Work out the finished part from the listing and answer in its coordinate system (mm). Round coordinates to 2 decimals unless told otherwise and drop trailing zeros. Answer in a Markdown table with one row per item.
```python
from build123d import *

# Parameters (mm, degrees)
SKETCH1_R           = 1.65
SKETCH1_R_2         = 4.5
SKETCH1_R_3         = 2.2
SKETCH1_R_4         = 1.15
SKETCH1_W           = 22
SKETCH1_H           = 43
SKETCH1_W_2         = 40
SKETCH1_H_2         = 12
BOSS_EXTRUDE1_DEPTH = 3
FILLET2_R           = 3
FILLET3_R           = 2
FILLET4_R           = 10
SKETCH2_W           = 40
SKETCH2_H           = 3
BOSS_EXTRUDE2_DEPTH = 3
SKETCH3_W           = 40
SKETCH3_H           = 3
CUT_EXTRUDE1_DEPTH  = 3
FILLET5_R           = 3


with BuildPart() as part:
    # Sketch1 → Boss-Extrude1 (new body)
    with BuildSketch(Plane.XY):
        with BuildLine():
            Line((-65.69, -25.08927508), (-65.69, -107.741221405))
            Line((-65.69, -107.741221405), (-40.69, -107.741221405))
            Line((-40.69, -107.741221405), (-40.69, -164.982205675))
            Line((-40.69, -164.982205675), (40.69, -164.982205675))
            Line((40.69, -164.982205675), (40.69, -107.741221405))
            Line((40.69, -107.741221405), (65.69, -107.741221405))
            Line((65.69, -107.741221405), (65.69, -25.08927508))
            Line((65.69, -25.08927508), (28.641763355, 5.396592354))
            Line((28.641763355, 5.396592354), (28.641763355, 14.771578959))
            ThreePointArc((28.641763355, 14.771578959), (36.853483101, 20.369604934), (30.2775665, 27.821286413))
            Line((30.2775665, 27.821286413), (30.2775665, 37.695580673))
            Line((30.2775665, 37.695580673), (9.5975665, 65.017794325))
            Line((9.5975665, 65.017794325), (-9.5975665, 65.017794325))
            Line((-9.5975665, 65.017794325), (-30.2775665, 37.695580673))
            Line((-30.2775665, 37.695580673), (-30.2775665, 27.821286413))
            ThreePointArc((-30.2775665, 27.821286413), (-36.853483101, 20.369604934), (-28.641763355, 14.771578959))
            Line((-28.641763355, 14.771578959), (-28.641763355, 5.396592354))
            Line((-28.641763355, 5.396592354), (-65.69, -25.08927508))
        make_face()
        with Locations((-30.2775665, 21.193907325)):
            Circle(SKETCH1_R, mode=Mode.SUBTRACT)
        with Locations((-29.8216785, -158.982205675)):
            Circle(SKETCH1_R, mode=Mode.SUBTRACT)
        with Locations((-52.692806, -67.094311675)):
            Circle(SKETCH1_R, mode=Mode.SUBTRACT)
        with Locations(Location((30.2775665, 21.193907325, 0), (0, 0, 180))):
            Circle(SKETCH1_R, mode=Mode.SUBTRACT)
        with Locations(Location((52.692806, -67.094311675, 0), (0, 0, 180))):
            Circle(SKETCH1_R, mode=Mode.SUBTRACT)
        with Locations(Location((29.8216785, -158.982205675, 0), (0, 0, 180))):
            Circle(SKETCH1_R, mode=Mode.SUBTRACT)
        with Locations((0, -18.982205675)):
            Circle(SKETCH1_R_2, mode=Mode.SUBTRACT)
        with Locations((-16.5, 29.107738598)):
            Circle(SKETCH1_R, mode=Mode.SUBTRACT)
        with Locations(Location((16.5, 29.107738598, 0), (0, 0, 180))):
            Circle(SKETCH1_R, mode=Mode.SUBTRACT)
        with Locations((-8, 58.607738598)):
            Circle(SKETCH1_R, mode=Mode.SUBTRACT)
        with Locations(Location((8, 58.607738598, 0), (0, 0, 180))):
            Circle(SKETCH1_R, mode=Mode.SUBTRACT)
        with Locations((5, 42.607738598)):
            Circle(SKETCH1_R_3, mode=Mode.SUBTRACT)
        with Locations(Location((-5, 42.607738598, 0), (0, 0, 180))):
            Circle(SKETCH1_R_3, mode=Mode.SUBTRACT)
        with Locations(Location((5, -7.392261402, 0), (0, 0, 180))):
            Circle(SKETCH1_R_3, mode=Mode.SUBTRACT)
        with Locations((-5, -7.392261402)):
            Circle(SKETCH1_R_3, mode=Mode.SUBTRACT)
        with Locations((-18.75, -160.982205675)):
            Circle(SKETCH1_R, mode=Mode.SUBTRACT)
        with Locations(Location((18.75, -160.982205675, 0), (0, 0, 180))):
            Circle(SKETCH1_R, mode=Mode.SUBTRACT)
        with Locations((18.75, -123.482205675)):
            Circle(SKETCH1_R, mode=Mode.SUBTRACT)
        with Locations(Location((-18.75, -123.482205675, 0), (0, 0, 180))):
            Circle(SKETCH1_R, mode=Mode.SUBTRACT)
        with Locations((21.5, -101.450066073)):
            Circle(SKETCH1_R_4, mode=Mode.SUBTRACT)
        with Locations(Location((-21.5, -101.450066073, 0), (0, 0, 180))):
            Circle(SKETCH1_R_4, mode=Mode.SUBTRACT)
        with Locations(Location((21.5, -32.450066073, 0), (0, 0, 180))):
            Circle(SKETCH1_R_4, mode=Mode.SUBTRACT)
        with Locations((-21.5, -32.450066073)):
            Circle(SKETCH1_R_4, mode=Mode.SUBTRACT)
        with Locations((0, 17.607738598)):
            Rectangle(SKETCH1_W, SKETCH1_H, mode=Mode.SUBTRACT)
        with Locations((0, -110.450066073)):
            Rectangle(SKETCH1_W_2, SKETCH1_H_2, mode=Mode.SUBTRACT)
        with BuildLine():
            Line((-27.5, -120.270969271), (-27.5, -140.086043436))
            ThreePointArc((-27.5, -140.086043436), (-30, -142.586043436), (-32.5, -140.086043436))
            Line((-32.5, -140.086043436), (-32.5, -120.270969271))
            ThreePointArc((-32.5, -120.270969271), (-30, -117.770969271), (-27.5, -120.270969271))
        make_face(mode=Mode.SUBTRACT)
        with BuildLine():
            Line((27.5, -120.270969271), (27.5, -140.086043436))
            ThreePointArc((27.5, -140.086043436), (30, -142.586043436), (32.5, -140.086043436))
            Line((32.5, -140.086043436), (32.5, -120.270969271))
            ThreePointArc((32.5, -120.270969271), (30, -117.770969271), (27.5, -120.270969271))
        make_face(mode=Mode.SUBTRACT)
        Polygon((20, -2.642677247), (20, -27.641099182), (45.282011772, -27.641099182), align=None, mode=Mode.SUBTRACT)
        Polygon((-20, -27.641099182), (-45.282011772, -27.641099182), (-20, -2.642677247), align=None, mode=Mode.SUBTRACT)
    extrude(amount=BOSS_EXTRUDE1_DEPTH)

    # Fillet2
    fillet2_edges = [part.edges().sort_by_distance(p)[0] for p in [
        (11, -3.892261402, 1.5),
        (11, 39.107738598, 1.5),
        (-11, 39.107738598, 1.5),
        (-11, -3.892261402, 1.5),
    ]]
    fillet(fillet2_edges, radius=FILLET2_R)

    # Fillet3
    fillet3_edges = [part.edges().sort_by_distance(p)[0] for p in [
        (45.282011772, -27.641099182, 1.5),
        (20, -2.642677247, 1.5),
        (20, -27.641099182, 1.5),
        (-20, -27.641099182, 1.5),
        (-20, -2.642677247, 1.5),
        (-45.282011772, -27.641099182, 1.5),
    ]]
    fillet(fillet3_edges, radius=FILLET3_R)

    # Fillet4
    fillet4_edges = [part.edges().sort_by_distance(p)[0] for p in [
        (65.69, -107.741221405, 1.5),
        (40.69, -107.741221405, 1.5),
        (40.69, -164.982205675, 1.5),
        (-40.69, -164.982205675, 1.5),
        (-40.69, -107.741221405, 1.5),
        (-65.69, -107.741221405, 1.5),
    ]]
    fillet(fillet4_edges, radius=FILLET4_R)

    # Sketch2 → Boss-Extrude2 (add)
    with BuildSketch(Plane.XZ.offset(104.450066073)):
        with Locations((0, 1.5)):
            Rectangle(SKETCH2_W, SKETCH2_H)
    extrude(amount=BOSS_EXTRUDE2_DEPTH)

    # Sketch3 → Cut-Extrude1 (cut)
    with BuildSketch(Plane(origin=(0, -116.450066073, 0), x_dir=(1, 0, 0), z_dir=(0, 1, 0))):
        with Locations((0, -1.5)):
            Rectangle(SKETCH3_W, SKETCH3_H)
    extrude(amount=-CUT_EXTRUDE1_DEPTH, mode=Mode.SUBTRACT)

    # Fillet5
    fillet5_edges = [part.edges().sort_by_distance(p)[0] for p in [
        (-20, -107.450066073, 1.5),
        (20, -107.450066073, 1.5),
        (-20, -119.450066073, 1.5),
        (20, -119.450066073, 1.5),
    ]]
    fillet(fillet5_edges, radius=FILLET5_R)


solid = part.part
```
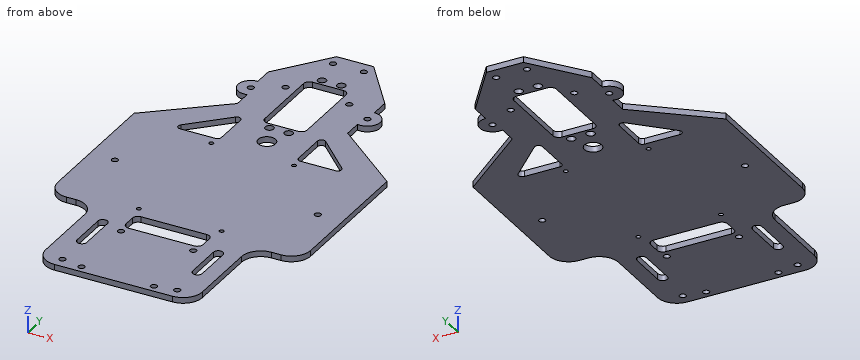
1. Consider line 1 along Y through (x, z) = (-36, 2.3); line 2 along Y through (x, z) = (0, 2.1); line 3 along X through (y, z) = (35.5, 2.2). Determine where each line is inside the solid, lowest interval first. Write a range as from..to.
Calculated:
| item | result |
|---|---|
| line 1 | y = -163.46..-27.64, -18.46..-0.66, 17.85..24.54 |
| line 2 | y = -164.98..-119.45, -107.45..-23.48, -14.48..-3.89, 39.11..65.02 |
| line 3 | x = -30.28..-11, 11..30.28 |
2. Given pin 1 (0.9 mm diameter, centred on y = 20.5, z = 2, fed in from +X); pin 2 (0.9 mm diameter, centred on y = -141.5, z = 1, fed in from -X); pin 3 (0.9 mm diameter, centred on y = -14, z = 1.5, fed in from -X), each flat-ended and moving along its own axis, determine where each tip first touches the part or whether it passes through.
Calculated:
| item | result |
|---|---|
| pin 1 | stops at x = 36.9 |
| pin 2 | stops at x = -40.69 |
| pin 3 | stops at x = -52.76 |
3. The part is cut by section A-A (z = 2.3). Count the separate pieces of the cut face and the enclosed holes in it, plus the area to 3 significant figures.
Calculated:
| item | result |
|---|---|
| separate pieces | 1 |
| enclosed holes | 29 |
| area | 19,000 mm² |
